The model under review builds one solid part; all positions refer to its coordinate system, in mm. A direction names the side the tool comes from. Give positions to 0.01 mm unless a question says otherwise; leave off trailing zeros. Order: outer loops, then holes, each group sorted by start corner. A loop starts at its lowest first (then second) coordinate and runs counter-clockwise, first axis right, second up.
```python
from build123d import *

# Parameters (mm, degrees)
SKETCH1_W                      = 42
SKETCH1_H                      = 145.161285219
BOSS_EXTRUDE1_DEPTH            = 5
BOSS_EXTRUDE2_DEPTH            = 5
SKETCH3_W                      = 5
SKETCH3_H                      = 27.999999523
BOSS_EXTRUDE3_DEPTH            = 81.000003815
F_5_5_5_5_DIAMETER_HOLE1_D     = 5.5
F_5_5_5_5_DIAMETER_HOLE2_D     = 5.5
F_5_5_5_5_DIAMETER_HOLE2_DEPTH = 5
F_5_5_5_5_DIAMETER_HOLE3_D     = 5.5
F_5_5_5_5_DIAMETER_HOLE3_DEPTH = 5
SKETCH10_W                     = 5
SKETCH10_H                     = 42
BOSS_EXTRUDE4_DEPTH            = 4.8


with BuildPart() as part:
    # Sketch1 → Boss-Extrude1 (new body)
    with BuildSketch(Plane(origin=(-5, 0, 0), x_dir=(0, -1, 0), z_dir=(-1, 0, 0))):
        with Locations((21, -72.58064261)):
            Rectangle(SKETCH1_W, SKETCH1_H)
    extrude(amount=-BOSS_EXTRUDE1_DEPTH)

    # Sketch2 → Boss-Extrude2 (add)
    with BuildSketch(Plane(origin=(0, 0, -150), x_dir=(-1, 0, 0), z_dir=(0, 0, -1))):
        Polygon((130, -43.400001526), (160, -43.400001526), (160, 0), (5, 0), (5, -27.999999523), (130, -27.999999523), align=None)
    extrude(amount=-BOSS_EXTRUDE2_DEPTH)

    # Sketch3 → Boss-Extrude3 (add)
    with BuildSketch(Plane.ZY.offset(5)):
        with Locations((-2.5, -13.999999762)):
            Rectangle(SKETCH3_W, SKETCH3_H)
    extrude(amount=BOSS_EXTRUDE3_DEPTH)

    # Ø5.5 (5.5) Diameter Hole1 (through all)
    with Locations(Plane.ZY.offset(5)):
        with Locations((-37.500000596, -22.500000199), (-25.000000199, -9.99999995), (-50.000000795, -9.99999995), (-62.500000795, -22.500000199), (-75.000000795, -9.99999995), (-87.500000795, -22.500000199), (-112.500000795, -22.500000199), (-100.000000795, -9.99999995), (-125.000000795, -9.99999995)):
            Hole(F_5_5_5_5_DIAMETER_HOLE1_D / 2)

    # Ø5.5 (5.5) Diameter Hole2
    with Locations(Plane.XY.offset(-145)):
        with Locations((-30.000000199, -9.99999995), (-42.500000397, -22.500000199), (-67.500000795, -22.500000199), (-55.000000795, -9.99999995), (-80.000001192, -9.99999995), (-92.500000795, -22.500000199), (-117.500000795, -22.500000199), (-105.000000795, -9.99999995), (-130.000003179, -9.99999995)):
            Hole(F_5_5_5_5_DIAMETER_HOLE2_D / 2, depth=F_5_5_5_5_DIAMETER_HOLE2_DEPTH)

    # Ø5.5 (5.5) Diameter Hole3
    with Locations(Plane(origin=(0, 0, -5), x_dir=(-1, 0, 0), z_dir=(0, 0, -1))):
        with Locations((80.50000151, -9.99999995), (68.000001113, -22.500000199), (43.000001113, -22.500000199), (55.500001113, -9.99999995), (30.500000119, -9.99999995)):
            Hole(F_5_5_5_5_DIAMETER_HOLE3_D / 2, depth=F_5_5_5_5_DIAMETER_HOLE3_DEPTH)

    # Sketch10 → Boss-Extrude4 (add)
    with BuildSketch(Plane(origin=(0, 0, -145.161285219), x_dir=(-1, 0, 0), z_dir=(0, 0, -1))):
        with Locations((2.5, -21)):
            Rectangle(SKETCH10_W, SKETCH10_H)
    extrude(amount=BOSS_EXTRUDE4_DEPTH)


solid = part.part
```
Item 1: Draft analysis for pull direction Z (two halves, no side actions). For faces 4 (the flat face through (-2, -21, -149.961)), 5 (the cylindrical face through (-2.47, -21.67, -90.12)), 6 (the flat face through (-45, -28, -3)), state which applies: released by +Z, released by -Z, zero draft, split by the parting line, or undercut.
Values found:
face 4: released by -Z
face 5: undercut
face 6: zero draft
Item 2: Clearance check with flat-ended pins moving along their axes: pin 1 Ø6.5 at (y, z) = (-22.5, -112.5) entering from -X; pin 2 Ø2.5 at (y, z) = (-11, -2) entering from -X; pin 3 Ø4 at (x, y) = (-3, -29) entering from -Z. State where each tip first meets the part, or that it passes through.
Values found:
pin 1: stops at x = -5
pin 2: stops at x = -86
pin 3: stops at z = -149.96
Item 3: Take a section at D-D (x = -150). Give the boundary of the cut face in (y, z).
Values found:
outline: (-43.4, -150) - (0, -150) - (0, -145) - (-43.4, -145) - close
Item 4: Take a section at B-B (z = -87.5). Give the boundary of the cut face in (x, y), and give its area (4 significant figures).
Values found:
outline: (-5, -42) - (0, -42) - (0, -25.25) - (-5, -25.25) - close; (-5, -19.75) - (0, -19.75) - (0, 0) - (-5, 0) - close
area: 182.5 mm2
Item 5: For line 1 (X direction, y = -22.5, z = -147.4); line 2 (Z direction, x = -39, y = -16); line 3 (Y direction, x = -55, z = -146.1), list the stretches that pass through material, from the lowest coordinate up.
Values found:
line 1: x = -160 to -120.25, -114.75 to -95.25, -89.75 to -70.25, -64.75 to -45.25, -39.75 to 0
line 2: z = -150 to -145, -5 to 0
line 3: y = -28 to -12.75, -7.25 to 0
Item 6: Take a section at C-C (x = -55). Give the boundary of the cut face in (y, z), and give its area (3 significant figures).
Values found:
outline: (-28, -150) - (-12.75, -150) - (-12.75, -145) - (-28, -145) - close; (-28, -5) - (-12.7, -5) - (-12.7, 0) - (-28, 0) - close; (-7.3, -5) - (0, -5) - (0, 0) - (-7.3, 0) - close; (-7.25, -150) - (0, -150) - (0, -145) - (-7.25, -145) - close
area: 225 mm2
Item 7: For faces 1 (the flat face through (-45, -14, -5)), 2 (the flat face through (-67, -28, -148)), 3 (the cylindrical face through (-43.358, -19.773, -2.465)), list the 3-axis set-ups (+Z, -Z, +X, -X, +Y, -Y) from which the entire face can be reached by the end or side of a thin tool; tool diameter is ignored.
Values found:
face 1: -X, +Y, -Y
face 2: +Z, -Z, -Y
face 3: +Z
Item 8: Take a section at A-A (x = -105). Give the boundary of the cut face in (y, z), and give its area (4 significant figures).
Values found:
outline: (-28, -150) - (-12.75, -150) - (-12.75, -145) - (-28, -145) - close; (-7.25, -150) - (0, -150) - (0, -145) - (-7.25, -145) - close
area: 112.5 mm2
